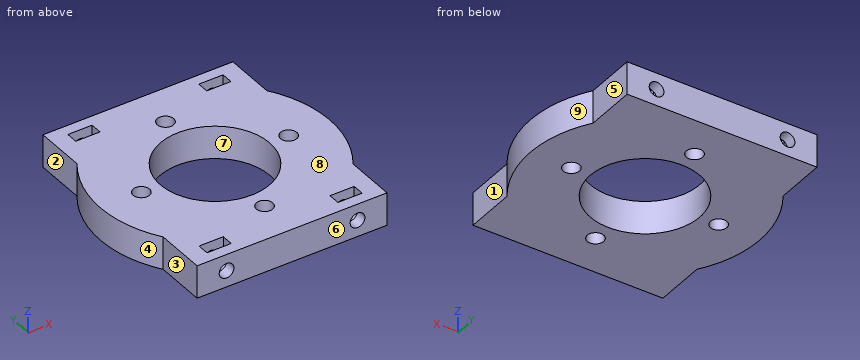
from build123d import *

# Parameters (mm, degrees)
CROQUIS1_R              = 16.7005
SALIENTE_EXTRUIR1_DEPTH = 5
CORTAR_EXTRUIR1_DEPTH   = 3.6
CROQUIS6_R              = 2.25
CORTAR_EXTRUIR2_DEPTH   = 10
CORTAR_EXTRUIR3_REACH   = 52.498
CROQUIS7_R              = 2.5


with BuildPart() as part:
    # Croquis1 → Saliente-Extruir1 (new, symmetric)
    with BuildSketch(Plane.XY):
        with BuildLine():
            Line((-29, 19.595917942), (-29, 35))
            Line((-29, 35), (29, 35))
            Line((29, 35), (29, 19.595917942))
            ThreePointArc((29, 19.595917942), (35, 0), (29, -19.595917942))
            Line((29, -19.595917942), (29, -35))
            Line((29, -35), (-29, -35))
            Line((-29, -35), (-29, -19.595917942))
            ThreePointArc((-29, -19.595917942), (-35, 0), (-29, 19.595917942))
        make_face()
        Circle(CROQUIS1_R, mode=Mode.SUBTRACT)
    extrude(amount=SALIENTE_EXTRUIR1_DEPTH, both=True)

    # Croquis5 → Cortar-Extruir1 (cut)
    with BuildSketch(Plane(origin=(0, 28, 0), x_dir=(1, 0, 0), z_dir=(0, 1, 0))):
        Polygon((-23.7, -2.136195996), (-23.7, -5), (-16.3, -5), (-16.3, -2.136195996), (-16.3, 2.136195996), (-20, 4.272391992), (-23.7, 2.136195996), align=None)
        Polygon((16.3, 2.136195996), (16.3, -2.136195996), (16.3, -5), (23.7, -5), (23.7, -2.136195996), (23.7, 2.136195996), (20, 4.272391992), align=None)
    cortar_extruir1 = extrude(amount=CORTAR_EXTRUIR1_DEPTH, mode=Mode.SUBTRACT)

    # Croquis6 → Cortar-Extruir2 (cut)
    with BuildSketch(Plane(origin=(0, 35, 0), x_dir=(1, 0, 0), z_dir=(0, 1, 0))):
        with Locations(Location((-20, 0, 0), (0, 0, 270))):
            Circle(CROQUIS6_R)
        with Locations(Location((20, 0, 0), (0, 0, 270))):
            Circle(CROQUIS6_R)
    cortar_extruir2 = extrude(amount=-CORTAR_EXTRUIR2_DEPTH, mode=Mode.SUBTRACT)

    # Simetría1: Cortar-Extruir1, Cortar-Extruir2 across plane
    add(cortar_extruir1.mirror(Plane.ZX), mode=Mode.SUBTRACT)
    add(cortar_extruir2.mirror(Plane.ZX), mode=Mode.SUBTRACT)

    # Croquis7 → Cortar-Extruir3 (cut, up to next)
    with BuildSketch(Plane.XY.offset(5), mode=Mode.PRIVATE) as cortar_extruir3_sk1:
        with Locations((0, 22.5)):
            Circle(CROQUIS7_R)
    cortar_extruir3_tool1 = extrude(cortar_extruir3_sk1.sketch, amount=-CORTAR_EXTRUIR3_REACH, mode=Mode.PRIVATE) & part.part
    # Croquis7 → Cortar-Extruir3 (cut, up to next)
    with BuildSketch(Plane.XY.offset(5), mode=Mode.PRIVATE) as cortar_extruir3_sk2:
        with Locations((22.5, 0)):
            Circle(CROQUIS7_R)
    cortar_extruir3_tool2 = extrude(cortar_extruir3_sk2.sketch, amount=-CORTAR_EXTRUIR3_REACH, mode=Mode.PRIVATE) & part.part
    # Croquis7 → Cortar-Extruir3 (cut, up to next)
    with BuildSketch(Plane.XY.offset(5), mode=Mode.PRIVATE) as cortar_extruir3_sk3:
        with Locations((0, -22.5)):
            Circle(CROQUIS7_R)
    cortar_extruir3_tool3 = extrude(cortar_extruir3_sk3.sketch, amount=-CORTAR_EXTRUIR3_REACH, mode=Mode.PRIVATE) & part.part
    # Croquis7 → Cortar-Extruir3 (cut, up to next)
    with BuildSketch(Plane.XY.offset(5), mode=Mode.PRIVATE) as cortar_extruir3_sk4:
        with Locations((-22.5, 0)):
            Circle(CROQUIS7_R)
    cortar_extruir3_tool4 = extrude(cortar_extruir3_sk4.sketch, amount=-CORTAR_EXTRUIR3_REACH, mode=Mode.PRIVATE) & part.part
    add(cortar_extruir3_tool1.solids().sort_by_distance((0, 22.5, 5))[0], mode=Mode.SUBTRACT)
    add(cortar_extruir3_tool2.solids().sort_by_distance((22.5, 0, 5))[0], mode=Mode.SUBTRACT)
    add(cortar_extruir3_tool3.solids().sort_by_distance((0, -22.5, 5))[0], mode=Mode.SUBTRACT)
    add(cortar_extruir3_tool4.solids().sort_by_distance((-22.5, 0, 5))[0], mode=Mode.SUBTRACT)


solid = part.part
Geometry check sheet. Reference: the model listing, model coordinates, mm. Face numbers are marked on the shaded views. A direction names the side the tool comes from. Coordinates: 2 decimals unless noted, no trailing zeros. Order: outer loops, then holes, each group sorted by start corner. A loop starts at its lowest first (then second) coordinate and runs counter-clockwise, first axis right, second up. Notation, with made-up numbers: (67.5, 67.25) - (113.5, 67.25) arc R24 cw to (113.5, 78.25) - close; hole circle Ø5 at (65.25, -26). An arc over 180 degrees is marked (long way). Answer in a Markdown table with one row per item. Add a question column.
1) Material ranges on line 1 along X through (y, z) = (-32.5, 0); line 2 along Y through (x, z) = (-22.5, -1.5); line 3 along Y through (x, z) = (0, -2.5), recorded low to high. Write a range as [from, to].
2) Release check for a two-part mould opening along Y. For the marked faces 6, 7, 8 and 9 record: +Y half, -Y half, draft (parallel to the pull), parting line (faces both ways), or undercut.
3) Set-up check for the marked faces 1, 2, 3, 4 and 5: record each of +Z, -Z, +X, -X, +Y, -Y from which the full face is reachable in a straight line by a thin tool's end or side.
4) Cross-section at A-A, the plane y = 22.5. Record the cut outline in (x, z).
5) Cross-section at D-D, the plane z = 4. State how many separate pieces and enclosed holes the cut face has, then the cut area to 3 significant figures.
6) Cross-section at B-B, the plane x = 0. Record the cut outline in (y, z).
7) Gauge pin test, flat ends, axial feed: P1, Ø4.5, axis at x = 0, y = 22.5, coming from the -Z side; P2, Ø1.3, axis at x = -19.5, z = -1, coming from the +Y side; P3, Ø1.1, axis at y = 30.5, z = 2.5, coming from the +X side; P4, Ø5, axis at y = -5, z = 1, coming from the +X side. Record the tip position at first contact, or that the pin passes through.
Check result:
| question | item | result |
|---|---|---|
| 1 | line 1 | x = [-29, -22.25], [-17.75, 17.75], [22.25, 29] |
| 1 | line 2 | y = [-35, -31.6], [-28, -2.5], [2.5, 28], [31.6, 35] |
| 1 | line 3 | y = [-35, -25], [-20, -16.7], [16.7, 20], [25, 35] |
| 2 | face 6 | -Y half |
| 2 | face 7 | undercut |
| 2 | face 8 | draft |
| 2 | face 9 | parting line |
| 3 | face 1 | +Z, -Z, +X, -Y |
| 3 | face 2 | +Z, -Z, -X, +Y |
| 3 | face 3 | +Z, -Z, -X, -Y |
| 3 | face 4 | +Z, -Z, -X |
| 3 | face 5 | +Z, -Z, +X, +Y |
| 4 | outline | (-29, -5) - (-2.5, -5) - (-2.5, 5) - (-29, 5) - close; (2.5, -5) - (29, -5) - (29, 5) - (2.5, 5) - close |
| 5 | separate pieces | 1 |
| 5 | enclosed holes | 9 |
| 5 | area | 3,320 mm² |
| 6 | outline | (-35, -5) - (-25, -5) - (-25, 5) - (-35, 5) - close; (-20, -5) - (-16.7, -5) - (-16.7, 5) - (-20, 5) - close; (16.7, -5) - (20, -5) - (20, 5) - (16.7, 5) - close; (25, -5) - (35, -5) - (35, 5) - (25, 5) - close |
| 7 | P1 | passes through |
| 7 | P2 | stops at y = 25 |
| 7 | P3 | stops at x = 29 |
| 7 | P4 | stops at x = 34.91 |
